from build123d import *

# Parameters (mm, degrees)
F0_W     = 127
F0_H     = 76.2
F1_DEPTH = 25.4
F2_R     = 6.35
F3_DEPTH = 25.401


with BuildPart() as f1:
    # F0 (on Top) → F1 (new body)
    with BuildSketch(Plane.XY):
        Rectangle(F0_W, F0_H)
    extrude(amount=F1_DEPTH)

    # F2 (on Top) → F3 (cut, through all)
    with BuildSketch(Plane.XY):
        with Locations((-48.03089, -27.837213)):
            Circle(F2_R)
        with Locations((44.281855, -27.837213)):
            Circle(F2_R)
        with Locations((42.659267, 23.51901)):
            Circle(F2_R)
        with Locations((-48.03089, 24.004152)):
            Circle(F2_R)
    extrude(amount=F3_DEPTH, mode=Mode.SUBTRACT)


solid = f1.part
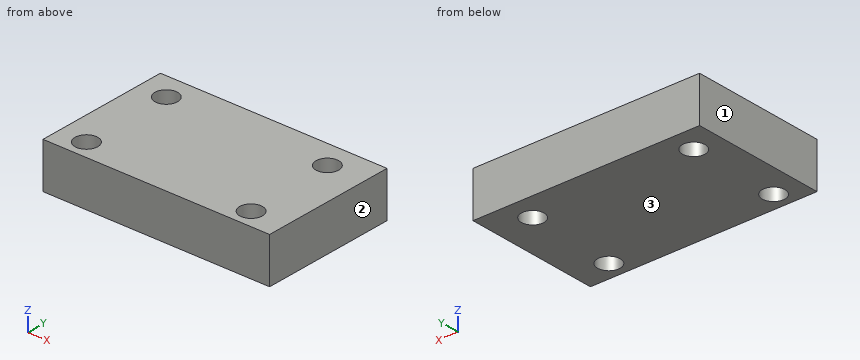
The model under review builds one solid part; all positions refer to its coordinate system, in mm. Face numbers are marked on the shaded views. Round coordinates to 2 decimals unless told otherwise and drop trailing zeros. Loops run counter-clockwise (first coordinate to the right, second up) from the corner with the lowest first, then second, coordinate; pieces in that order, holes last. Notation, with made-up numbers: M -3.75,-26 L 29.25,-26 A26 ccw 29.25,10 Z; hole C 35,-14.75 d6. An arc over 180 degrees is marked long. Answer as CSV lines item,"result".
1. We need section B-B (y = 26.5). Give the boundary of the cut face in (x, z), plus the area to 3 significant figures.
Outcome:
outline,"M -63.5,0 L -53.87,0 L -53.87,25.4 L -63.5,25.4 Z; M -42.19,0 L 37.05,0 L 37.05,25.4 L -42.19,25.4 Z; M 48.27,0 L 63.5,0 L 63.5,25.4 L 48.27,25.4 Z"
area,"2,640 mm2"
2. Insertion check: pin 1 Ø7.5 at (x, y) = (-48.03, -27.84) entering from -Z. The pin has a flat end and moves straight along its axis. Give the tip position at first contact, or say it passes through.
Outcome:
pin 1,"passes through"
3. To check wall thickness, follow L1, parallel to X at y = -27.5, z = 23.75; L2, parallel to X at y = 20.5, z = 9.5; L3, parallel to Y at x = 37, z = 9.5. State the ranges of each line that lie inside material, in increasing order. Write a range as [from, to].
Outcome:
L1,"x = [-63.5, -54.37], [-41.69, 37.94], [50.62, 63.5]"
L2,"x = [-63.5, -53.33], [-42.74, 37.07], [48.25, 63.5]"
L3,"y = [-38.1, 20.64], [26.4, 38.1]"
4. We need section C-C (z = 18). Give the boundary of the cut face in (x, y).
Outcome:
outline,"M -63.5,-38.1 L 63.5,-38.1 L 63.5,38.1 L -63.5,38.1 Z; hole C -48.03,-27.84 d12.7; hole C -48.03,24 d12.7; hole C 42.66,23.52 d12.7; hole C 44.28,-27.84 d12.7"
5. We need section A-A (x = -49). Give the boundary of the cut face in (y, z), plus the area to 3 significant figures.
Outcome:
outline,"M -38.1,0 L -34.11,0 L -34.11,25.4 L -38.1,25.4 Z; M -21.56,0 L 17.73,0 L 17.73,25.4 L -21.56,25.4 Z; M 30.28,0 L 38.1,0 L 38.1,25.4 L 30.28,25.4 Z"
area,"1,300 mm2"
6. Draft analysis for pull direction X (two halves, no side actions). For the marked faces 1, 2 and 3, state which applies: pulls with the +X half, pulls with the -X half, needs draft (parallel to the pull), parting line crosses it, or undercut.
Outcome:
face 1,"pulls with the -X half"
face 2,"pulls with the +X half"
face 3,"needs draft"
